from build123d import *

# Parameters (mm, degrees)
SKETCH1_R               = 11.25
BOSS_EXTRUDE1_DEPTH     = 4
SKETCH2_W               = 2
SKETCH2_H               = 2.8
CUT_EXTRUDE2_DEPTH      = 18.808003819
CIRPATTERN1_START       = -4
CIRPATTERN1_DEPTH       = 8
CUT_EXTRUDE3_DEPTH      = 18.751760477
CUT_EXTRUDE3_DEPTH_BACK = 18.751760477
SKETCH4_R               = 2


# Read off the part's stored shape, not the designer's step: CirPattern1
with BuildPart() as part:
    # Sketch1 → Boss-Extrude1 (new, symmetric)
    with BuildSketch(Plane.XY):
        Circle(SKETCH1_R)
    extrude(amount=BOSS_EXTRUDE1_DEPTH, both=True)

    # Sketch2 → Cut-Extrude2 (cut, symmetric)
    with BuildSketch(Plane.XY.offset(4)):
        with Locations((0, 9.805467416)):
            Rectangle(SKETCH2_W, SKETCH2_H)
    extrude(amount=CUT_EXTRUDE2_DEPTH, both=True, mode=Mode.SUBTRACT)


with BuildPart() as cut_extrude2_kept_piece:
    # of the separate pieces the step leaves, the one the design keeps (cut_extrude2_pieces_kept)
    add(part.part.solids().sort_by_distance((1, 8.405467416, 4))[0])

    # CirPattern1 outline → CirPattern1 (cut)
    with BuildSketch(Plane.XY.offset(CIRPATTERN1_START)):
        with BuildLine():
            Line((1, -8.405467416), (-1, -8.405467416))
            Line((-1, -8.405467416), (-1, -11.205467416))
            ThreePointArc((-1, -11.205467416), (0, -11.25), (1, -11.205467416))
            Line((1, -11.205467416), (1, -8.405467416))
        make_face()
        with BuildLine():
            Line((4.140512654, 7.382955874), (5.212026264, 9.969818566))
            ThreePointArc((5.212026264, 9.969818566), (4.305188614, 10.393644741), (3.364267199, 10.73518543))
            Line((3.364267199, 10.73518543), (2.292753589, 8.148322739))
            Line((2.292753589, 8.148322739), (4.140512654, 7.382955874))
        make_face()
        with BuildLine():
            Line((6.65066979, 5.236456227), (8.630568777, 7.216355215))
            ThreePointArc((8.630568777, 7.216355215), (7.954951289, 7.954951289), (7.216355215, 8.630568777))
            Line((7.216355215, 8.630568777), (5.236456227, 6.65066979))
            Line((5.236456227, 6.65066979), (6.65066979, 5.236456227))
        make_face()
        with BuildLine():
            Line((8.148322739, 2.292753589), (10.73518543, 3.364267199))
            ThreePointArc((10.73518543, 3.364267199), (10.393644741, 4.305188614), (9.969818565, 5.212026264))
            Line((9.969818565, 5.212026264), (7.382955874, 4.140512654))
            Line((7.382955874, 4.140512654), (8.148322739, 2.292753589))
        make_face()
        with BuildLine():
            Line((8.405467416, -1), (11.205467416, -1))
            ThreePointArc((11.205467416, -1), (11.25, 0), (11.205467416, 1))
            Line((11.205467416, 1), (8.405467416, 1))
            Line((8.405467416, 1), (8.405467416, -1))
        make_face()
        with BuildLine():
            Line((7.382955874, -4.140512654), (9.969818565, -5.212026264))
            ThreePointArc((9.969818565, -5.212026264), (10.393644741, -4.305188614), (10.73518543, -3.364267199))
            Line((10.73518543, -3.364267199), (8.148322739, -2.292753589))
            Line((8.148322739, -2.292753589), (7.382955874, -4.140512654))
        make_face()
        with BuildLine():
            Line((5.236456227, -6.65066979), (7.216355215, -8.630568777))
            ThreePointArc((7.216355215, -8.630568777), (7.954951288, -7.954951288), (8.630568777, -7.216355215))
            Line((8.630568777, -7.216355215), (6.65066979, -5.236456227))
            Line((6.65066979, -5.236456227), (5.236456227, -6.65066979))
        make_face()
        with BuildLine():
            Line((2.292753589, -8.148322739), (3.364267199, -10.73518543))
            ThreePointArc((3.364267199, -10.73518543), (4.305188614, -10.393644741), (5.212026264, -9.969818565))
            Line((5.212026264, -9.969818565), (4.140512654, -7.382955874))
            Line((4.140512654, -7.382955874), (2.292753589, -8.148322739))
        make_face()
        with BuildLine():
            ThreePointArc((-3.364267199, 10.73518543), (-4.305188614, 10.393644741), (-5.212026264, 9.969818566))
            Line((-5.212026264, 9.969818566), (-4.140512654, 7.382955874))
            Line((-4.140512654, 7.382955874), (-2.292753589, 8.148322739))
            Line((-2.292753589, 8.148322739), (-3.364267199, 10.73518543))
        make_face()
        with BuildLine():
            ThreePointArc((-7.216355215, 8.630568777), (-7.954951289, 7.954951289), (-8.630568777, 7.216355215))
            Line((-8.630568777, 7.216355215), (-6.65066979, 5.236456227))
            Line((-6.65066979, 5.236456227), (-5.236456227, 6.65066979))
            Line((-5.236456227, 6.65066979), (-7.216355215, 8.630568777))
        make_face()
        with BuildLine():
            ThreePointArc((-9.969818565, 5.212026264), (-10.393644741, 4.305188614), (-10.73518543, 3.364267199))
            Line((-10.73518543, 3.364267199), (-8.148322739, 2.292753589))
            Line((-8.148322739, 2.292753589), (-7.382955874, 4.140512654))
            Line((-7.382955874, 4.140512654), (-9.969818565, 5.212026264))
        make_face()
        with BuildLine():
            ThreePointArc((-11.205467416, 1), (-11.25, 0), (-11.205467416, -1))
            Line((-11.205467416, -1), (-8.405467416, -1))
            Line((-8.405467416, -1), (-8.405467416, 1))
            Line((-8.405467416, 1), (-11.205467416, 1))
        make_face()
        with BuildLine():
            ThreePointArc((-10.73518543, -3.364267199), (-10.393644741, -4.305188614), (-9.969818565, -5.212026264))
            Line((-9.969818565, -5.212026264), (-7.382955874, -4.140512654))
            Line((-7.382955874, -4.140512654), (-8.148322739, -2.292753589))
            Line((-8.148322739, -2.292753589), (-10.73518543, -3.364267199))
        make_face()
        with BuildLine():
            ThreePointArc((-8.630568777, -7.216355215), (-7.954951288, -7.954951288), (-7.216355215, -8.630568777))
            Line((-7.216355215, -8.630568777), (-5.236456227, -6.65066979))
            Line((-5.236456227, -6.65066979), (-6.65066979, -5.236456227))
            Line((-6.65066979, -5.236456227), (-8.630568777, -7.216355215))
        make_face()
        with BuildLine():
            ThreePointArc((-5.212026264, -9.969818565), (-4.305188614, -10.393644741), (-3.364267199, -10.73518543))
            Line((-3.364267199, -10.73518543), (-2.292753589, -8.148322739))
            Line((-2.292753589, -8.148322739), (-4.140512654, -7.382955874))
            Line((-4.140512654, -7.382955874), (-5.212026264, -9.969818565))
        make_face()
    extrude(amount=CIRPATTERN1_DEPTH, mode=Mode.SUBTRACT)

    # Sketch4 → Cut-Extrude3 (cut, two sides: drawn at the far end of the back side and taken through both)
    with BuildSketch(Plane.XY.offset(4).offset(-CUT_EXTRUDE3_DEPTH_BACK)):
        Circle(SKETCH4_R)
    extrude(amount=CUT_EXTRUDE3_DEPTH + CUT_EXTRUDE3_DEPTH_BACK, mode=Mode.SUBTRACT)


solid = cut_extrude2_kept_piece.part
Design review of the part built by this model. Coordinates are the model's own, in mm. A direction names the side the tool comes from. Coordinates: 2 decimals unless noted, no trailing zeros. Loops run counter-clockwise (first coordinate to the right, second up) from the corner with the lowest first, then second, coordinate; pieces in that order, holes last. Notation, with made-up numbers: M 66,17.5 L 72,17.5 A27 cw 72,38.5 Z; hole C 31.5,-37 d4. An arc over 180 degrees is marked long. Answer as CSV lines item,"result".
Item 1: Add section A-A on y = 0. State the section outline as (x, z) points, plus the area to 3 significant figures.
Answer list:
outline,"M -8.41,-4 L -2,-4 L -2,4 L -8.41,4 Z; M 2,-4 L 8.41,-4 L 8.41,4 L 2,4 Z"
area,"102 mm²"
Item 2: Add section C-C on y = -3. State the section outline as (x, z) points, plus the area to 3 significant figures.
Answer list:
outline,"M -10.84,-4 L -9.86,-4 L -9.86,4 L -10.84,4 Z; M -7.86,-4 L 7.86,-4 L 7.86,4 L -7.86,4 Z; M 9.86,-4 L 10.84,-4 L 10.84,4 L 9.86,4 Z"
area,"141 mm²"
Item 3: For P1, Ø0.8, axis at y = -10, z = 0, coming from the -X side; P2, Ø3, axis at x = 8.5, z = 2.5, coming from the -Y side; P3, Ø0.6, axis at x = -0.5, z = -1.5, coming from the -Y side, all flat-tipped, find the tip position at first contact; note any pin that passes through.
Answer list:
P1,"x = -5.87"
P2,"y = -8.81"
P3,"y = -8.41"
Item 4: For probe 1 along Y at (x, z) = (0, -2.25); probe 2 along X at (y, z) = (-8.5, 2), list the stretches that pass through material, from the lowest coordinate up.
Answer list:
probe 1,"-8.41 to -2, 2 to 8.41"
probe 2,"-7.09 to -4.6, -2.44 to -1, 1 to 2.44, 4.6 to 7.09"
Item 5: Machinability: for faces 1 (the face through (1, -10, 0)), 2 (the face through (-10, -1, 0)), 3 (the face through (5.953, -5.934, -0.056)), 4 (the face through (0, 8.405, 0)), 5 (the face through (8.405, 0, 0)), which of the approach directions +Z, -Z, +X, -X, +Y, -Y give a long, thin tool a straight path to every point of the face, cutting with its end or side? Answer none if there is none.
Answer list:
face 1,"+Z, -Z, -Y"
face 2,"+Z, -Z, -X"
face 3,"+Z, -Z"
face 4,"+Z, -Z, +Y"
face 5,"+Z, -Z, +X"
Item 6: Add section D-D on x = -4.5. State the section outline as (y, z) points, plus the area to 3 significant figures.
Answer list:
outline,"M -8.25,-4 L 8.25,-4 L 8.25,4 L -8.25,4 Z"
area,"132 mm²"
Item 7: The part is to be moulded in two halves that separate along X. For faces 6 (the face through (-8.405, 0, 0)), 7 (the face through (6.24, -9.36, 0.06)), 8 (the face through (3.204, 7.771, -0.056)), say which applies: pulls with the +X half, pulls with the -X half, needs draft (parallel to the pull), parting line crosses it, or undercut.
Answer list:
face 6,"pulls with the -X half"
face 7,"pulls with the +X half"
face 8,"undercut"
Item 8: Add section B-B on x = 1.5. State the section outline as (y, z) points, plus the area to 3 significant figures.
Answer list:
outline,"M -11.15,-4 L -1.32,-4 L -1.32,4 L -11.15,4 Z; M 1.32,-4 L 11.15,-4 L 11.15,4 L 1.32,4 Z"
area,"157 mm²"
